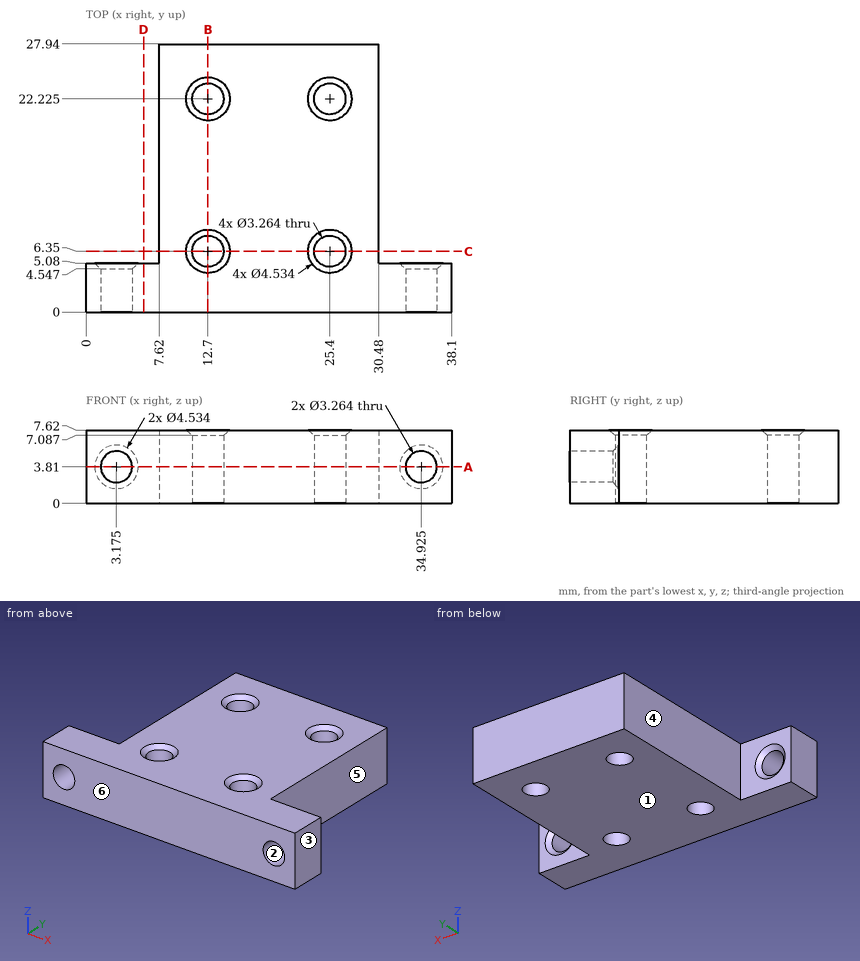
Answer from the drawing. Dimensions are ordinates in mm from the lowest x, y and z of the part. A direction names the side the tool comes from. Give positions to 0.01 mm unless a question says otherwise; leave off trailing zeros. Loops run counter-clockwise (first coordinate to the right, second up) from the corner with the lowest first, then second, coordinate; pieces in that order, holes last. Notation, with made-up numbers: (65, 29.5) - (121, 29.5) arc R6 cw to (121, 38.5) - close; hole circle Ø10 at (72, -35.75). An arc over 180 degrees is marked (long way). Write each question's results on one line, items separated by ' | '.
1. Find section D-D, the plane x = 6. Write down the section's boundary in (y, z), then the cut area to 3 significant figures.
Resolved:
outline: (0, 0) - (5.08, 0) - (5.08, 7.62) - (0, 7.62) - close | area: 38.7 mm^2
2. Which of the six approach directions +Z, -Z, +X, -X, +Y, -Y give full straight-line access (tool end or side, diameter ignored) to the marked faces 4, 5 and 6?
Resolved:
face 4: +Z, -Z, -X, +Y | face 5: +Z, -Z, +X, +Y | face 6: +Z, -Z, +X, -X, -Y
3. Find section A-A, the plane z = 3.81. Count the separate pieces of the cut face and the enclosed holes in it, then the cut area to 3 significant figures.
Resolved:
separate pieces: 3 | enclosed holes: 4 | area: 649 mm^2
4. Find section B-B, the plane x = 12.7. Write down the section's boundary in (y, z).
Resolved:
outline: (0, 0) - (4.72, 0) - (4.72, 7.09) - (4.08, 7.62) - (0, 7.62) - close; (7.98, 0) - (20.59, 0) - (20.59, 7.09) - (19.96, 7.62) - (8.62, 7.62) - (7.98, 7.09) - close; (23.86, 0) - (27.94, 0) - (27.94, 7.62) - (24.49, 7.62) - (23.86, 7.09) - close
5. For a pull along Z with two mould halves and no side action, classify the marked faces 1, 2 and 3 as +Z half, -Z half, draft (parallel to the pull), parting line (faces both ways), or undercut.
Resolved:
face 1: -Z half | face 2: undercut | face 3: draft
6. Find section C-C, the plane y = 6.35. Write down the section's boundary in (x, z), then the cut area to 3 significant figures.
Resolved:
outline: (7.62, 0) - (11.07, 0) - (11.07, 7.09) - (10.43, 7.62) - (7.62, 7.62) - close; (14.33, 0) - (23.77, 0) - (23.77, 7.09) - (23.13, 7.62) - (14.97, 7.62) - (14.33, 7.09) - close; (27.03, 0) - (30.48, 0) - (30.48, 7.62) - (27.67, 7.62) - (27.03, 7.09) - close | area: 124 mm^2
7. Flat-ended cylindrical pins translate along their axes: P1, Ø2.5, axis at x = 25.4, y = 22.225, coming from the +Z side; P2, Ø2, axis at y = 22, z = 4, coming from the +X side; P3, Ø4, axis at x = 3.175, z = 3.81, coming from the +Y side; P4, Ø2, axis at y = 21, z = 2.5, coming from the -X side. Find the tip coordinate at first contact, or state that the pin passes through.
Resolved:
P1: passes through | P2: stops at x = 30.48 | P3: stops at y = 4.86 | P4: stops at x = 7.62
8. Consider probe 1 along X at (y, z) = (6.35, 5); probe 2 along Y at (x, z) = (12.7, 5.25); probe 3 along Z at (x, y) = (4, 4). Determine where each line is inside the solid, lowest interval first. Write a range as from..to.
Resolved:
probe 1: x = 7.62..11.07, 14.33..23.77, 27.03..30.48 | probe 2: y = 0..4.72, 7.98..20.59, 23.86..27.94 | probe 3: z = 0..2.4, 5.22..7.62
